Source: CAD feature listing. Evaluate the final solid. Frame: model axes, mm. Face numbers are marked on the shaded views. A direction names the side the tool comes from. Coordinates: 2 decimals unless noted, no trailing zeros. Write each loop counter-clockwise with the first axis right and the second up, starting at its lowest first coordinate (ties: lowest second). Pieces come first, ordered by that corner, then holes. Notation, with made-up numbers: (32, 77) - (66, 77) arc R16 cw to (66, 98) - close; hole circle Ø9 at (-10, -35). An arc over 180 degrees is marked (long way). One line per item, written item: value.
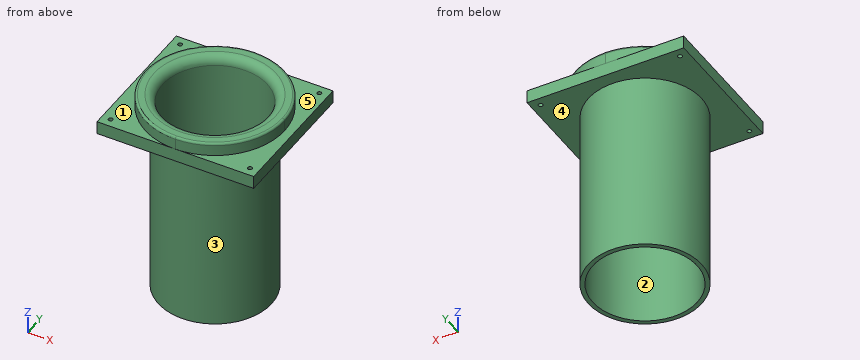
from build123d import *

# Parameters (mm, degrees)
F0_R     = 3.175
F1_DEPTH = 19.05
F0_R_2   = 82.55
F0_R_3   = 76.2
F2_DEPTH = 38.1
F3_DEPTH = 266.7
F4_R     = 12.7
F5_R     = 3.175


with BuildPart() as f1:
    # F0 (on Top) → F1 (new body)
    with BuildSketch(Plane.XY):
        with BuildLine():
            Line((0, 203.2), (0, 0))
            Line((0, 0), (114.3, 0))
            ThreePointArc((114.3, 0), (12.7, 101.6), (114.3, 203.2))
            Line((114.3, 203.2), (0, 203.2))
        make_face()
        with Locations((12.7, 12.7)):
            Circle(F0_R, mode=Mode.SUBTRACT)
        with Locations((12.7, 190.5)):
            Circle(F0_R, mode=Mode.SUBTRACT)
    extrude(amount=F1_DEPTH)



with BuildPart() as f1b:
    # F0 (on Top) → F1, piece 2 (new body)
    with BuildSketch(Plane.XY):
        with BuildLine():
            ThreePointArc((215.9, 101.6), (186.1420489686, 29.7579510314), (114.3, 0))
            Line((114.3, 0), (228.6, 0))
            Line((228.6, 0), (228.6, 203.2))
            Line((228.6, 203.2), (114.3, 203.2))
            ThreePointArc((114.3, 203.2), (186.1420489686, 173.4420489686), (215.9, 101.6))
        make_face()
        with Locations((215.9, 12.7)):
            Circle(F0_R, mode=Mode.SUBTRACT)
        with Locations((215.9, 190.5)):
            Circle(F0_R, mode=Mode.SUBTRACT)
    extrude(amount=F1_DEPTH)


with BuildPart() as f1_1:
    add(f1.part)

    add(f1b.part)  # F2 merges F1b
    # F0 (on Top) → F2 (join)
    with BuildSketch(Plane.XY):
        with BuildLine():
            ThreePointArc((114.3, 203.2), (12.7, 101.6), (114.3, 0))
            ThreePointArc((114.3, 0), (186.1420489686, 29.7579510314), (215.9, 101.6))
            ThreePointArc((215.9, 101.6), (186.1420489686, 173.4420489686), (114.3, 203.2))
        make_face()
        with Locations((114.3, 101.6)):
            Circle(F0_R_2, mode=Mode.SUBTRACT)
        with Locations((114.3, 101.6)):
            Circle(F0_R_2)
        with Locations((114.3, 101.6)):
            Circle(F0_R_3, mode=Mode.SUBTRACT)
    extrude(amount=F2_DEPTH)

    # F0 (on Top) → F3 (join)
    with BuildSketch(Plane.XY):
        with Locations((114.3, 101.6)):
            Circle(F0_R_2)
        with Locations((114.3, 101.6)):
            Circle(F0_R_3, mode=Mode.SUBTRACT)
    extrude(amount=-F3_DEPTH)

    # F4
    f4_edges = [f1_1.edges().sort_by_distance(p)[0] for p in [
        (38.1, 101.6, 38.1),
    ]]
    fillet(f4_edges, radius=F4_R)

    # F5
    f5_edges = [f1_1.edges().sort_by_distance(p)[0] for p in [
        (114.3, 0, 38.1),
    ]]
    fillet(f5_edges, radius=F5_R)


solid = f1_1.part
1) Draft query along X for the marked faces 1, 2 and 3. Return one class per face: released by +X, released by -X, zero draft, split by the parting line, or undercut.
Values found:
face 1: zero draft
face 2: undercut
face 3: split by the parting line
2) Material intervals for line 1 (Y direction, x = 12.7, z = 13) (3 decimals); line 2 (X direction, y = 190.5, z = 8.25) (3 decimals); line 3 (X direction, y = 104.5, z = -65.5), sorted ascending.
Values found:
line 1: 0 to 9.525, 15.875 to 187.325, 193.675 to 203.2
line 2: 0 to 9.525, 15.875 to 212.725, 219.075 to 228.6
line 3: 31.8 to 38.16, 190.44 to 196.8
3) Section query A-A on z = -177. Output: boundary loops of the cut face in (x, y).
Values found:
outline: circle Ø165.1 at (114.3, 101.6); hole circle Ø152.4 at (114.3, 101.6)
4) Contact query for flat-ended pins moving along their axis: P1, Ø4, axis at x = 12.7, y = 12.7, coming from the +Z side; P2, Ø3, axis at x = 87.5, z = -179.5, coming from the +Y side; P3, Ø1, axis at x = 95.5, z = -122.5, coming from the -Y side; P4, Ø10, axis at x = 190, z = -82.5, coming from the +Y side. Output: stop coordinate, or through.
Values found:
P1: through
P2: y = 180.18
P3: y = 21.1
P4: y = 144.21
5) Reachability of the marked faces 4 and 5 from +Z, -Z, +X, -X, +Y, -Y: full face, straight path, thin tool, end or side. Return the list, or none.
Values found:
face 4: -Z
face 5: +Z, +X
